```python
from build123d import *

# Parameters (mm, degrees)
SKETCH_1_W      = 120
SKETCH_1_H      = 74
SKETCH_1_R      = 1.6
EXTRUDE_2_DEPTH = 1.6
SKETCH_2_W      = 105.5
SKETCH_2_H      = 67.2
EXTRUDE_3_DEPTH = 3.1


with BuildPart() as part:
    # 草图1 → 凸台-拉伸2 (new body)
    with BuildSketch(Plane(origin=(0, 0, 0), x_dir=(1, 0, 0), z_dir=(0, 1, 0))):
        Rectangle(SKETCH_1_W, SKETCH_1_H)
        with Locations(Location((-56.8, 33.8, 0), (0, 0, 270))):
            Circle(SKETCH_1_R, mode=Mode.SUBTRACT)
        with Locations(Location((-56.8, -33.8, 0), (0, 0, 90))):
            Circle(SKETCH_1_R, mode=Mode.SUBTRACT)
        with Locations(Location((56.8, -33.8, 0), (0, 0, 270))):
            Circle(SKETCH_1_R, mode=Mode.SUBTRACT)
        with Locations(Location((56.8, 33.8, 0), (0, 0, 90))):
            Circle(SKETCH_1_R, mode=Mode.SUBTRACT)
    extrude(amount=EXTRUDE_2_DEPTH)

    # 草图2 → 凸台-拉伸3 (add)
    with BuildSketch(Plane.XZ):
        Rectangle(SKETCH_2_W, SKETCH_2_H)
    extrude(amount=EXTRUDE_3_DEPTH)


solid = part.part
```
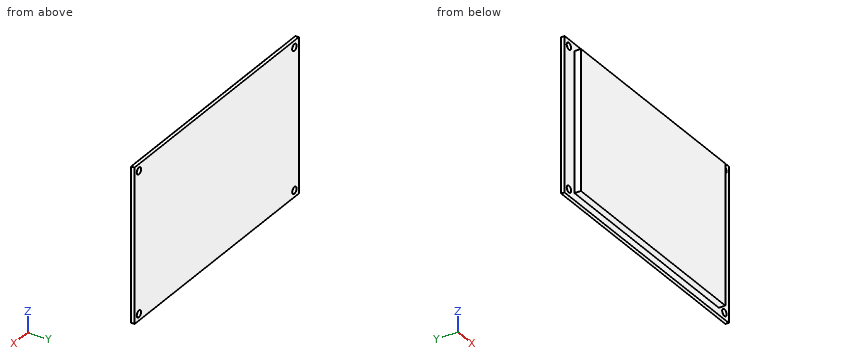
Can you work these out from the model? Positions are in its coordinate system, mm. Coordinates: 2 decimals unless noted, no trailing zeros. Loops run counter-clockwise (first coordinate to the right, second up) from the corner with the lowest first, then second, coordinate; pieces in that order, holes last.
Item 1: I'm going to push flat-ended pins straight in: pin 1 (1.9 mm diameter, centred on x = 56.8, z = 33.8, fed in from -Y) (3 decimals); pin 2 (1.6 mm diameter, centred on x = 23, y = -1, fed in from -Z); pin 3 (1.5 mm diameter, centred on x = 35.5, y = -1, fed in from +Z); pin 4 (1 mm diameter, centred on y = -2, z = -19.5, fed in from +X). Where does each tip first touch, or does it pass through?
Answers below:
pin 1: passes through
pin 2: stops at z = -33.6
pin 3: stops at z = 33.6
pin 4: stops at x = 52.75
Item 2: Please list where these lines run through material, in increasing order: L1, parallel to X at y = 0.65, z = -33.8; L2, parallel to Z at x = -27, y = -0.65; L3, parallel to X at y = -0.85, z = 10.
Answers below:
L1: x = -60 to -58.4, -55.2 to 55.2, 58.4 to 60
L2: z = -33.6 to 33.6
L3: x = -52.75 to 52.75
Item 3: Suppose I cut it at A-A (x = 56.8). Please give me the cut outline in (y, z), then the cut area to 3 significant figures.
Answers below:
outline: (0, -37) - (1.6, -37) - (1.6, -35.4) - (0, -35.4) - close; (0, -32.2) - (1.6, -32.2) - (1.6, 32.2) - (0, 32.2) - close; (0, 35.4) - (1.6, 35.4) - (1.6, 37) - (0, 37) - close
area: 108 mm2
Item 4: Suppose I cut it at B-B (z = -5.5). Please give me the cut outline in (x, y).
Answers below:
outline: (-60, 0) - (-52.75, 0) - (-52.75, -3.1) - (52.75, -3.1) - (52.75, 0) - (60, 0) - (60, 1.6) - (-60, 1.6) - close
